Geometry check sheet. Reference: the model listing, model coordinates, mm. Face numbers are marked on the shaded views. A direction names the side the tool comes from. Round coordinates to 2 decimals unless told otherwise and drop trailing zeros. Loops run counter-clockwise (first coordinate to the right, second up) from the corner with the lowest first, then second, coordinate; pieces in that order, holes last. Notation, with made-up numbers: (22.25, -3) - (67.25, -3) arc R16 cw to (67.25, 11) - close; hole circle Ø4 at (42, -4.5). An arc over 180 degrees is marked (long way). Answer as CSV lines item,"result". Start each with the question number.
1) Cross-section at A-A on x = 0. Record the boundary of the cut face in (y, z), and give its area (3 significant figures).
2) Cross-section at C-C on y = -5.5. Record the boundary of the cut face in (x, z).
3) Cross-section at B-B on z = 0. Record the boundary of the cut face in (x, y).
4) Cross-section at D-D on x = -413. Record the boundary of the cut face in (y, z), and give its area (3 significant figures).
5) Thickness scan on line 1 along Z through (x, y) = (0, 2.3); line 2 along Z through (x, y) = (-337, -1.5); line 3 along X through (y, z) = (1.5, -1). Record the ranges inside material, lowest first.
6) Access from +Z, -Z, +X, -X, +Y, -Y to the whole of each face (thin tool, end or side, straight path). Record for the marked faces 1 and 2.
7) Depth check by flat-ended pin: P1, Ø3, axis at x = -48, z = 47.5, coming from the -Y side. Enter the tip coordinate at first touch or a pass-through.
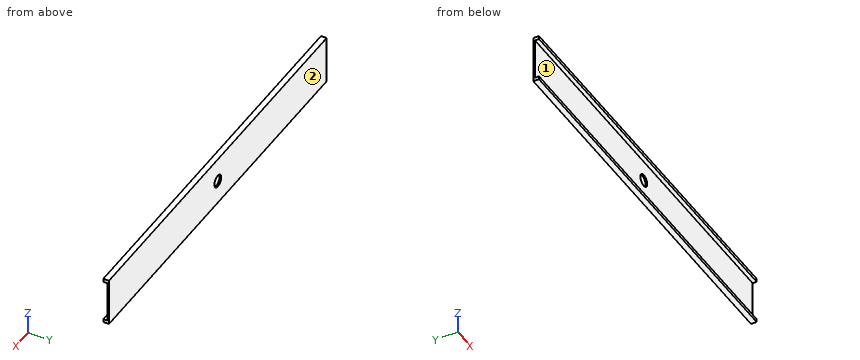
from build123d import *

# Parameters (mm, degrees)
SKETCH1_W               = 960
SKETCH1_H               = 120
BOSS_EXTRUDE1_DEPTH     = 4
CUT_EXTRUDE1_DEPTH      = 24
CUT_EXTRUDE1_DEPTH_BACK = 13
SKETCH2_R               = 15
SKETCH3_W               = 960
SKETCH3_H               = 8.349001696
BOSS_EXTRUDE2_DEPTH     = 10
SKETCH4_W               = 960
SKETCH4_H               = 8.113720408
BOSS_EXTRUDE3_DEPTH     = 10


with BuildPart() as part:
    # Sketch1 → Boss-Extrude1 (new body)
    with BuildSketch(Plane(origin=(0, 0, 0), x_dir=(1, 0, 0), z_dir=(0, 1, 0))):
        Rectangle(SKETCH1_W, SKETCH1_H)
    extrude(amount=BOSS_EXTRUDE1_DEPTH)

    # Sketch2 → Cut-Extrude1 (cut, two sides: drawn at the far end of the back side and taken through both)
    with BuildSketch(Plane(origin=(0, 4, 0), x_dir=(1, 0, 0), z_dir=(0, 1, 0)).offset(-CUT_EXTRUDE1_DEPTH_BACK)):
        with Locations(Location((0, 0, 0), (0, 0, 270))):
            Circle(SKETCH2_R)
    extrude(amount=CUT_EXTRUDE1_DEPTH + CUT_EXTRUDE1_DEPTH_BACK, mode=Mode.SUBTRACT)

    # Sketch3 → Boss-Extrude2 (add)
    with BuildSketch(Plane.XZ):
        with Locations((0, 55.825499152)):
            Rectangle(SKETCH3_W, SKETCH3_H)
    extrude(amount=BOSS_EXTRUDE2_DEPTH)

    # Sketch4 → Boss-Extrude3 (add)
    with BuildSketch(Plane.XZ):
        with Locations((0, -55.943139796)):
            Rectangle(SKETCH4_W, SKETCH4_H)
    extrude(amount=BOSS_EXTRUDE3_DEPTH)


solid = part.part
Answer block:
1,outline,"(-10, -60) - (4, -60) - (4, -15) - (0, -15) - (0, -51.89) - (-10, -51.89) - close; (-10, 51.65) - (0, 51.65) - (0, 15) - (4, 15) - (4, 60) - (-10, 60) - close"
1,area,"525 mm^2"
2,outline,"(-480, -60) - (480, -60) - (480, -51.89) - (-480, -51.89) - close; (-480, 51.65) - (480, 51.65) - (480, 60) - (-480, 60) - close"
3,outline,"(-480, 0) - (-15, 0) - (-15, 4) - (-480, 4) - close; (15, 0) - (480, 0) - (480, 4) - (15, 4) - close"
4,outline,"(-10, -60) - (4, -60) - (4, 60) - (-10, 60) - (-10, 51.65) - (0, 51.65) - (0, -51.89) - (-10, -51.89) - close"
4,area,"645 mm^2"
5,line 1,"z = -60 to -15, 15 to 60"
5,line 2,"z = -60 to -51.89, 51.65 to 60"
5,line 3,"x = -480 to -14.97, 14.97 to 480"
6,face 1,"+X, -X, -Y"
6,face 2,"+Z, -Z, +X, -X, +Y"
7,P1,"stops at y = 0"
